Autodesk Inventor part; units mm, degrees
ref_plane "YZ Plane" through (0, 0, 0) normal (1, 0, 0) x (0, 1, 0)
ref_plane "XZ Plane" through (0, 0, 0) normal (0, 1, 0) x (-1, 0, 0)
ref_plane "XY Plane" through (0, 0, 0) normal (0, 0, 1) x (1, 0, 0)
sketch "Skizze1" plane through (0, 0, 0) normal (0, 0, 1) x (1, 0, 0)
  line L0 (-16.3284, 0) -> (97.9706, 0)
  line L1 (0, -8.5) -> (0, 51)
  line L2 (0, 0) -> (0, 25)
  line L3 (0, 25) -> (57.5, 25)
  line L4 (62.5, 30) -> (62.5, 39.5)
  line L5 (77.5, 39.5) -> (77.5, 25)
  line L6 (57.5, 5) -> (30, 5)
  line L7 (25, 0) -> (25, 0)
  arc A0 (57.5, 5) -> (77.5, 25) centre (57.5, 25) ccw
  arc A1 (57.5, 25) -> (62.5, 30) centre (57.5, 30) ccw
  arc A2 (30, 5) -> (25, 0) centre (30, 0) ccw
  arc A3 (62.5, 39.5) -> (65.5, 42.5) centre (62.5, 42.5) ccw
  arc A4 (74.5, 42.5) -> (77.5, 39.5) centre (77.5, 42.5) ccw
  line L8 (65.5, 42.5) -> (74.5, 42.5)
  point P0 (62.5, 25)
  point P1 (77.5, 5)
  point P2 (25, 5)
  dimension "d0" = 77.5
  dimension "d3" = 25
  dimension "d4" = 5
  dimension "d5" = 25
  dimension "d11" = 20
  dimension "d12" = 5
  dimension "d19" = 15
  dimension "d21" = 42.5
  dimension "d22" = 3
  dimension "d23" = 3
extrude "Grundkörper" add sketch "Skizze1" along normal blind 5
sketch "Skizze2" plane through (0, 0, 5) normal (0, 0, 1) x (1, 0, 0)
  line L0 (0, -8.5) -> (0, 51)
  line L1 (-15.5, 0) -> (93, 0)
  line L2 (30, 5) -> (57.5, 5)
  circle A0 centre (11.5, 2.5) radius 1.6
  circle A1 centre (17, 14.5) radius 8
  circle A2 centre (21.5, 2.5) radius 1.6
  circle A3 centre (37, 15.5) radius 7
  circle A4 centre (54, 17.5) radius 5
  circle A5 centre (67, 22.5) radius 4
  circle A6 centre (70, 35) radius 2.5
  point P0 (0, 0)
  dimension "d24" = 11.5
  dimension "d25" = 10
  dimension "d26" = 2.5
  dimension "d27" = 2.5
  dimension "d28" = 14.5
  dimension "d29" = 17
  dimension "d30" = 10.5
  dimension "d31" = 37
  dimension "d32" = 12.5
  dimension "d33" = 54
  dimension "d34" = 17.5
  dimension "d35" = 67
  dimension "d36" = 70
  dimension "d37" = 35
  dimension "d38" = 16
  dimension "d39" = 3.2
  dimension "d40" = 3.2
  dimension "d41" = 14
  dimension "d42" = 10
  dimension "d43" = 8
  dimension "d44" = 5
extrude "Extrusion2" cut sketch "Skizze2" against normal through all
sketch "Skizze3" plane through (0, 0, 0) normal (-1, 0, 0) x (0, 0, 1)
  line L0 (0, -8.5) -> (0, 51)
  line L1 (-1, 0) -> (6, 0)
  point P0 (0, 0)
  point P1 (2.5, 10)
  dimension "d47" = 10
  dimension "d48" = 2.5
hole "Bohrung1" at (0, 10, 2.5) direction (1, 0, 0) diameter 2.459 depth 7 tip angle 118
sketch "Skizze4" plane through (65.5, 42.5, 0) normal (0, 1, 0) x (1, 0, 0)
  line L0 (-81, 0) -> (27.5, 0)
  line L1 (12, 0) -> (12, -5)
  point P0 (-65.5, 0)
  point P1 (4.5, -2.5)
  dimension "d56" = 7.5
  dimension "d57" = 2.5
hole "Bohrung2" at (70, 42.5, 2.5) direction (0, -1, 0) diameter 2.459 end up to surface
properties part number "Lagerarm"
Source: CAD feature listing. Evaluate the final solid. Frame: model axes, mm. A direction names the side the tool comes from. Give positions to 0.01 mm unless a question says otherwise; leave off trailing zeros. Loops run counter-clockwise (first coordinate to the right, second up) from the corner with the lowest first, then second, coordinate; pieces in that order, holes last. Notation, with made-up numbers: (72, -9.5) -> (106, -9.5) arc R19 cw to (106, 17.5) -> close; hole circle Ø1 at (81, 8.5). An arc over 180 degrees is marked (long way). Use a Markdown table: item, result. Add a question column.
(1) Section query C-C (x = 11.5). Output: boundary loops of the cut face in (y, z).
(2) Section query A-A (x = 54). Output: boundary loops of the cut face in (y, z).
(3) Pull-direction query (X, two-part tool) for faces 4 (the face through (12, 0, 2)), 5 (the face through (0, 12, 2)), 6 (the face through (9.9, 2.57, 2.54)), 7 (the face through (52.92, 12.62, 2.54)); classes: +X half, -X half, draft (parallel to the pull), parting line (faces both ways), or undercut.
(4) Access query for faces 1 (the face through (3.549, 10.471, 3.636)), 2 (the face through (44, 5, 2)), 3 (the face through (70.815, 23.701, 2.535)). Directions: +Z, -Z, +X, -X, +Y, -Y. A direction counts if a zero-diameter tool reaches every point of the face in a straight line with its end or side. Return the directions, or none.
(5) Ray query, line 1 (Y direction, x = 11.5, z = 2.95); line 2 (Y direction, x = 21.5, z = 2.4); line 3 (X direction, y = 19.5, z = 3.8) (3 decimals). Return the intervals inside material, ascending.
(6) First-contact query: pin 1 Ø1.5 at (x, z) = (26.5, 1.5) entering from +Y; pin 2 Ø2 at (x, z) = (70, 2.5) entering from -Y; pin 3 Ø2.5 at (x, z) = (44.5, 2) entering from -Y. Flat tips, straight axial feed; report the tip coordinate or a pass-through.
(7) Section query D-D (y = 2.5). Output: boundary loops of the cut face in (x, z).
(8) Section query B-B (y = 35). Output: boundary loops of the cut face in (x, z).
Checked values:
| question | item | result |
|---|---|---|
| 1 | outline | (0, 0) -> (0.9, 0) -> (0.9, 5) -> (0, 5) -> close; (4.1, 0) -> (8.69, 0) -> (8.69, 5) -> (4.1, 5) -> close; (20.31, 0) -> (25, 0) -> (25, 5) -> (20.31, 5) -> close |
| 2 | outline | (5, 0) -> (12.5, 0) -> (12.5, 5) -> (5, 5) -> close; (22.5, 0) -> (25, 0) -> (25, 5) -> (22.5, 5) -> close |
| 3 | face 4 | draft |
| 3 | face 5 | -X half |
| 3 | face 6 | undercut |
| 3 | face 7 | undercut |
| 4 | face 1 | -X |
| 4 | face 2 | +Z, -Z, +X, -Y |
| 4 | face 3 | +Z, -Z |
| 5 | line 1 | 0 to 0.9, 4.1 to 8.69, 20.31 to 25 |
| 5 | line 2 | 0 to 0.9, 4.1 to 7.89, 21.11 to 25 |
| 5 | line 3 | 0 to 10.755, 23.245 to 31.255, 42.745 to 49.417, 58.583 to 64.354, 69.646 to 76.729 |
| 6 | pin 1 | y = 25 |
| 6 | pin 2 | y = 8.64 |
| 6 | pin 3 | y = 5 |
| 7 | outline | (0, 0) -> (9.9, 0) -> (9.9, 5) -> (0, 5) -> close; (13.1, 0) -> (19.9, 0) -> (19.9, 5) -> (13.1, 5) -> close; (23.1, 0) -> (25.67, 0) -> (25.67, 5) -> (23.1, 5) -> close |
| 8 | outline | (62.5, 0) -> (67.5, 0) -> (67.5, 5) -> (62.5, 5) -> close; (72.5, 0) -> (77.5, 0) -> (77.5, 5) -> (72.5, 5) -> close |
